Work out the finished part from the listing and answer in its coordinate system (mm). Give positions to 0.01 mm unless a question says otherwise; leave off trailing zeros. Loops run counter-clockwise (first coordinate to the right, second up) from the corner with the lowest first, then second, coordinate; pieces in that order, holes last. Notation, with made-up numbers: (39.25, -22.75) -> (87.25, -22.75) arc R9 ccw to (87.25, -17.75) -> close; hole circle Ø4 at (-19.5, 66.25). An arc over 180 degrees is marked (long way). Answer as CSV lines item,"result". Start each with the question number.
1. Find section B-B, the plane z = 1.3. Count the separate pieces of the cut face and the enclosed holes in it, and give its area (3 significant figures).
2. Find section C-C, the plane x = 33.8. Give the vertices of the cut face in (y, z) (3 decimals), and give its area (3 significant figures).
3. Find section D-D, the plane y = 40. Give the vertices of the cut face in (x, z).
4. Determine the mould class of faces 1 (the face through (-27.02, -19.56, 1.42)), 2 (the face through (47.69, -15.02, 1.38)), 3 (the face through (-1, -10, 0)) for opening direction Y: +Y half, -Y half, draft (parallel to the pull), parting line (faces both ways), or undercut.
5. Find section A-A, the plane y = 2.3. Give the vertices of the cut face in (x, z) (3 decimals), and give its area (3 significant figures).
6. Flat-ended cylindrical pins translate along their axes: pin 1 Ø3 at (x, y) = (-10.49, -10.49) entering from -Z; pin 2 Ø1 at (y, z) = (-15.5, 1) entering from +X. Find the tip coordinate at first contact, or state that the pin passes through.
7. Find the intervals of material crossed by line 1 along Y through (x, z) = (0, 0.65); line 2 along Y through (x, z) = (-28, 1.45) (3 decimals); line 3 along Y through (x, z) = (14, 2.2), in increasing order.
Autodesk Inventor part; units mm, degrees
ref_plane "YZ Plane" through (0, 0, 0) normal (1, 0, 0) x (0, 1, 0)
ref_plane "XZ Plane" through (0, 0, 0) normal (0, 1, 0) x (-1, 0, 0)
ref_plane "XY Plane" through (0, 0, 0) normal (0, 0, 1) x (1, 0, 0)
sketch "Sketch1" plane through (0, 0, 0) normal (0, 0, 1) x (1, 0, 0)
  circle A0 centre (0, 0) radius 50
  dimension "d0" = 100
extrude "Extrusion1" add sketch "Sketch1" along normal blind 2.8
sketch "Sketch2" plane through (0, 0, 2.8) normal (0, 0, 1) x (1, 0, 0)
  circle A0 centre (0, 0) radius 50
  circle A1 centre (0, 0) radius 5
  dimension "d3" = 10
extrude "Extrusion2" cut sketch "Sketch2" against normal through all contours A1
sketch "Sketch3" plane through (0, 0, 2.8) normal (0, 0, 1) x (1, 0, 0)
  circle A0 centre (0, 0) radius 5
  line L0 (-70, 0) -> (70, 0)
  line L1 (0, -70) -> (0, 70)
  circle A1 centre (0, 14.84) radius 1
  circle A2 centre (-10.4935, 10.4935) radius 1
  circle A3 centre (-14.84, 0) radius 1
  circle A4 centre (-10.4935, -10.4935) radius 1
  circle A5 centre (0, -14.84) radius 1
  circle A6 centre (10.4935, -10.4935) radius 1
  circle A7 centre (14.84, 0) radius 1
  circle A8 centre (10.4935, 10.4935) radius 1
  circle A9 centre (-28, 2.3) radius 1.825
  circle A10 centre (-28, -21.1) radius 1.825
  circle A11 centre (33.8, -21.1) radius 1.825
  circle A12 centre (33.8, 2.3) radius 1.825
  dimension "d6" = 2
  dimension "d7" = 14.84
  dimension "d10" = 360
extrude "Extrusion3" cut sketch "Sketch3" against normal through all contours A5 L1 | L1 A5 | A3 L0 | L0 A3 | A1 L1 | L1 A1 | A7 L0 | L0 A7 | A2 | A4 | A6 | A8 | A9 | A10 | A11 | A12
properties part number "Acrylic_rotationServoTray"
Resolved:
1,separate pieces,"1"
1,enclosed holes,"13"
1,area,"7,710 mm^2"
2,outline,"(-36.845, 0) -> (-22.925, 0) -> (-22.925, 2.8) -> (-36.845, 2.8) -> close; (-19.275, 0) -> (0.475, 0) -> (0.475, 2.8) -> (-19.275, 2.8) -> close; (4.125, 0) -> (36.845, 0) -> (36.845, 2.8) -> (4.125, 2.8) -> close"
2,area,"186 mm^2"
3,outline,"(-30, 0) -> (30, 0) -> (30, 2.8) -> (-30, 2.8) -> close"
4,face 1,"undercut"
4,face 2,"parting line"
4,face 3,"draft"
5,outline,"(-49.947, 0) -> (-29.825, 0) -> (-29.825, 2.8) -> (-49.947, 2.8) -> close; (-26.175, 0) -> (-4.44, 0) -> (-4.44, 2.8) -> (-26.175, 2.8) -> close; (4.44, 0) -> (31.975, 0) -> (31.975, 2.8) -> (4.44, 2.8) -> close; (35.625, 0) -> (49.947, 0) -> (49.947, 2.8) -> (35.625, 2.8) -> close"
5,area,"234 mm^2"
6,pin 1,"stops at z = 0"
6,pin 2,"stops at x = 47.7"
7,line 1,"y = -50 to -15.84, -13.84 to -5, 5 to 13.84, 15.84 to 50"
7,line 2,"y = -41.425 to -22.925, -19.275 to 0.475, 4.125 to 41.425"
7,line 3,"y = -48 to -0.54, 0.54 to 48"
